Autodesk Inventor part; units mm, degrees
ref_plane "YZ Plane" through (0, 0, 0) normal (1, 0, 0) x (0, 1, 0)
ref_plane "XZ Plane" through (0, 0, 0) normal (0, 1, 0) x (-1, 0, 0)
ref_plane "XY Plane" through (0, 0, 0) normal (0, 0, 1) x (1, 0, 0)
sketch "Sketch1" plane through (0, 0, 0) normal (0, 0, 1) x (1, 0, 0)
  line L0 (-23.512, 105) -> (23.512, 105)
  line L1 (23.512, 105) -> (23.512, -105)
  line L2 (23.512, -105) -> (-23.512, -105)
  line L3 (-23.512, -105) -> (-23.512, 105)
  line L4 (-23.512, 105) -> (23.512, -105) construction
  line L5 (23.512, 105) -> (-23.512, -105) construction
  line L6 (-24.712, 106.2) -> (24.712, 106.2)
  line L7 (24.712, 106.2) -> (24.712, -106.2)
  line L8 (24.712, -106.2) -> (-24.712, -106.2)
  line L9 (-24.712, -106.2) -> (-24.712, 106.2)
  line L10 (-24.712, 106.2) -> (24.712, -106.2) construction
  line L11 (24.712, 106.2) -> (-24.712, -106.2) construction
  line L12 (23.512, -105) -> (24.712, -105)
  line L13 (-23.512, -105) -> (-24.712, -105)
  point P0 (0, 0)
  dimension "d0" = 47.024
  dimension "d1" = 210
  dimension "d2" = 1.2
  dimension "d3" = 1.2
extrude "Extrusion1" add sketch "Sketch1" along normal blind 64 contours L3 L13 L9 L6 L7 L12 L1 L0
sketch "Sketch2" plane through (0, 0, 64) normal (0, 0, 1) x (1, 0, 0)
  line L0 (23.512, -105) -> (24.712, -105)
  line L1 (24.712, -105) -> (24.712, 106.2)
  line L2 (24.712, 106.2) -> (-24.712, 106.2)
  line L3 (-24.712, 106.2) -> (-24.712, -105)
  line L4 (-24.712, -105) -> (-23.512, -105)
  line L5 (-23.512, -105) -> (-23.512, 105)
  line L6 (-23.512, 105) -> (23.512, 105)
  line L7 (23.512, 105) -> (23.512, -105)
  circle A0 centre (-29.712, -66.5359) radius 1.85
  line L8 (-24.712, -105) -> (-26.712, -105)
  line L9 (-26.712, -105) -> (-26.712, -75)
  line L10 (-32.712, -61.5359) -> (-32.712, -71.5359)
  line L11 (-32.712, -71.5359) -> (-26.712, -75)
  line L12 (-32.712, -61.5359) -> (-26.712, -58.0718)
  line L13 (-26.712, -75) -> (-26.712, -58.0718) construction
  line L14 (-32.712, 8.4641) -> (-26.712, 11.9282)
  line L15 (-32.712, 8.4641) -> (-32.712, -1.5359)
  line L16 (-32.712, -1.5359) -> (-26.712, -5)
  line L17 (-26.712, -5) -> (-26.712, 11.9282) construction
  circle A1 centre (-29.712, 3.4641) radius 1.85
  line L18 (-32.712, 78.4641) -> (-26.712, 81.9282)
  line L19 (-32.712, 78.4641) -> (-32.712, 68.4641)
  line L20 (-32.712, 68.4641) -> (-26.712, 65)
  line L21 (-26.712, 65) -> (-26.712, 81.9282) construction
  circle A2 centre (-29.712, 73.4641) radius 1.85
  line L22 (-26.712, -58.0718) -> (-26.712, -5)
  line L23 (-26.712, 11.9282) -> (-26.712, 65)
  line L24 (-26.712, 81.9282) -> (-26.712, 106.2)
  line L25 (-26.712, 106.2) -> (-24.712, 106.2)
  point P0 (0, 0)
  point P1 (-32.712, -66.5359)
  point P2 (-32.712, 3.4641)
  point P3 (-32.712, 73.4641)
  dimension "d6" = 3.7
  dimension "d7" = 5
  dimension "d8" = 3
  dimension "d9" = 10
  dimension "d10" = 60
  dimension "d11" = 60
  dimension "d12" = 30
  dimension "d13" = 2
  dimension "d16" = 70
extrude "Extrusion2" add sketch "Sketch2" against normal blind 3 contours L3 L8 L9 L11 L10 L12 L22 L16 L15 L14 L23 L20 L19 L18 L24 L25
mirror "Mirror1" about plane through (0, 0, 0) normal (1, 0, 0) of "Extrusion2"
equation "\"d3\" = d2"
equation "\"d11\" = d10"
properties part number "Drag Chain Cover" material "ABS Plastic"
For this review, take the finished solid that the model builds, in its own axes (mm). A direction names the side the tool comes from. Coordinates: 2 decimals unless noted, no trailing zeros. Write each loop counter-clockwise with the first axis right and the second up, starting at its lowest first coordinate (ties: lowest second). Pieces come first, ordered by that corner, then holes.
(1) Add section A-A on y = 29.5. Give the boundary of the cut face in (x, z).
(2) Add section C-C on x = -11. Give the boundary of the cut face in (y, z).
(3) Add section B-B on z = 33. Give the boundary of the cut face in (x, y).
(4) The part is to be moulded in two halves that separate along X. For faces 5 (the face through (-29.754, 10.172, 62.521)), 6 (the face through (29.67, -59.78, 62.52)), 7 (the face through (-31.56, 3.55, 62.52)), say which applies: +X half, -X half, draft (parallel to the pull), parting line (faces both ways), or undercut.
(5) For pin 1 Ø5 at (x, z) = (22.5, 44) entering from -Y; pin 2 Ø2.5 at (y, z) = (50.5, 62) entering from -X; pin 3 Ø1 at (y, z) = (-58.5, 8.5) entering from -X; pin 4 Ø3.5 at (y, z) = (38.5, 62) entering from +X, all flat-tipped, find the tip position at first contact; note any pin that passes through.
(6) Wall thickness on probe 1 along X at (y, z) = (34, 55); probe 2 along Y at (x, z) = (6, 13); probe 3 along Z at (x, y) = (-26.5, -5): over which ranges is each line inside the solid? List them lowest first.
(7) Tool access review of faces 1 (the face through (-23.512, -1, 32)), 2 (the face through (29.67, -3.29, 62.52)), 3 (the face through (-27, 2, 61)), 4 (the face through (24.712, 2, 30)): name each direction out of +Z, -Z, +X, -X, +Y, -Y from which nothing blocks a thin tool from reaching the whole face with its end or side.
Answer sheet:
1. outline: (-26.71, 61) - (-24.71, 61) - (-24.71, 0) - (-23.51, 0) - (-23.51, 64) - (-26.71, 64) - close; (23.51, 0) - (24.71, 0) - (24.71, 61) - (26.71, 61) - (26.71, 64) - (23.51, 64) - close
2. outline: (105, 0) - (106.2, 0) - (106.2, 64) - (105, 64) - close
3. outline: (-24.71, -105) - (-23.51, -105) - (-23.51, 105) - (23.51, 105) - (23.51, -105) - (24.71, -105) - (24.71, 106.2) - (-24.71, 106.2) - close
4. face 5: -X half
4. face 6: +X half
4. face 7: undercut
5. pin 1: stops at y = -105
5. pin 2: stops at x = -26.71
5. pin 3: stops at x = -24.71
5. pin 4: stops at x = 26.71
6. probe 1: x = -24.71 to -23.51, 23.51 to 24.71
6. probe 2: y = 105 to 106.2
6. probe 3: z = 61 to 64
7. face 1: +Z, -Z, -Y
7. face 2: +Z, -Z, +X
7. face 3: -Z, -X, +Y, -Y
7. face 4: -Z, +X, +Y, -Y
